Input: dimensioned drawing with shaded views. Units: mm. Origin: part minimum x, y, z. A direction names the side the tool comes from. Round coordinates to 2 decimals unless told otherwise and drop trailing zeros. Write each loop counter-clockwise with the first axis right and the second up, starting at its lowest first coordinate (ties: lowest second). Pieces come first, ordered by that corner, then holes. Notation, with made-up numbers: M 30,-24.75 L 75,-24.75 A19 ccw 75,-10.75 Z; hole C 66.25,-39 d10. An arc over 180 degrees is marked long. Put each result on its own line as item: value. Start each with the question number.
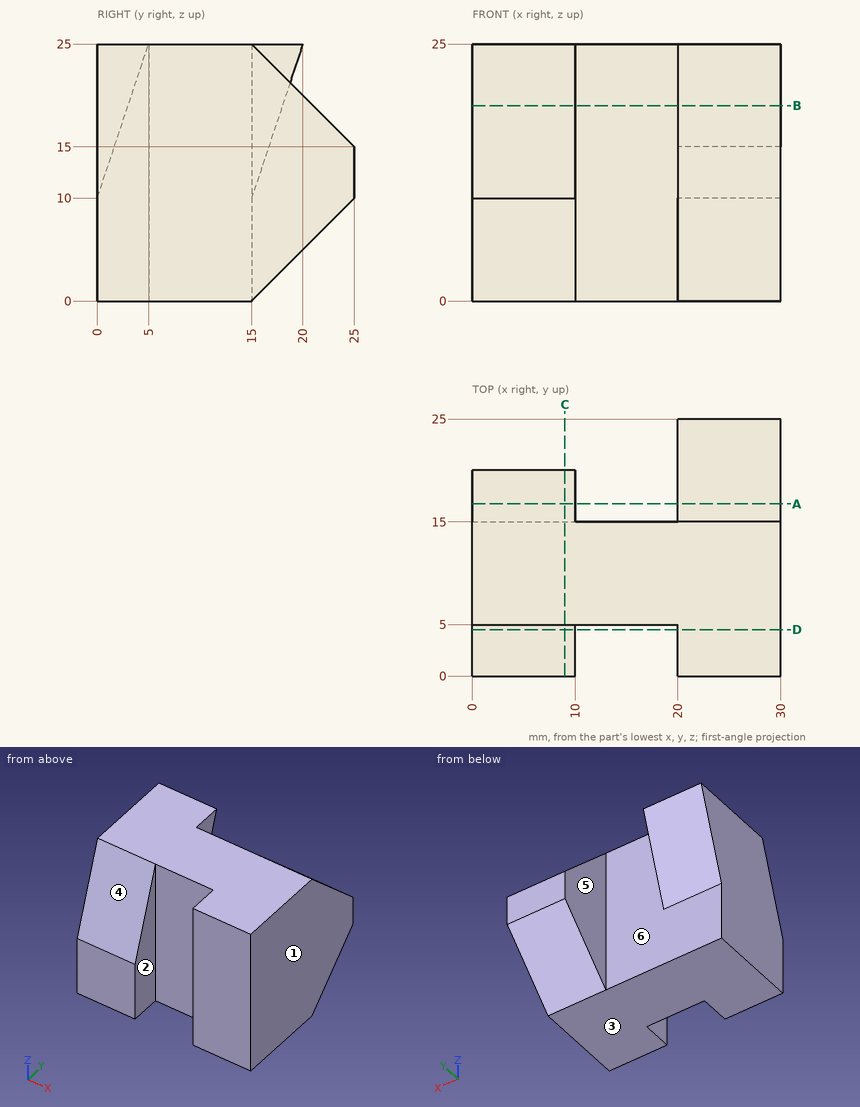
1) Section A-A, the plane y = 16.75. Output: boundary loops of the cut face in (x, z).
2) Section C-C, the plane x = 9. Output: boundary loops of the cut face in (y, z).
3) First-contact query: pin 1 (1 mm diameter, centred on x = 8, z = 22, fed in from +Y). Flat tip, straight axial feed; report the tip coordinate or a pass-through.
4) Section B-B, the plane z = 19. Output: boundary loops of the cut face in (x, y), and give its area (3 significant figures).
5) Ray query, probe 1 along Y at (x, z) = (11.5, 12.5); probe 2 along Z at (x, y) = (24, 18.75); probe 3 along Y at (x, z) = (5.75, 23). Return the intervals inside material, ascending.
6) Draft query along X for the marked faces 1, 2 and 3. Return one class per face: +X half, -X half, draft (parallel to the pull), parting line (faces both ways), or undercut.
7) Section D-D, the plane y = 4.5. Output: boundary loops of the cut face in (x, z).
8) Access query for the marked faces 4, 5 and 6. Directions: +Z, -Z, +X, -X, +Y, -Y. A direction counts if a zero-diameter tool reaches every point of the face in a straight line with its end or side. Return the directions, or none.
Solved:
1. outline: M 0,15.25 L 10,15.25 L 10,25 L 0,25 Z; M 20,1.75 L 30,1.75 L 30,23.25 L 20,23.25 Z
2. outline: M 0,0 L 15,0 L 15,10 L 20,25 L 5,25 L 0,10 Z
3. pin 1: stops at y = 19.17
4. outline: M 0,3 L 10,3 L 10,5 L 20,5 L 20,0 L 30,0 L 30,21 L 20,21 L 20,15 L 10,15 L 10,18 L 0,18 Z
4. area: 460 mm2
5. probe 1: y = 5 to 15
5. probe 2: z = 3.75 to 21.25
5. probe 3: y = 4.33 to 19.33
6. face 1: +X half
6. face 2: undercut
6. face 3: draft
7. outline: M 0,0 L 10,0 L 10,23.5 L 0,23.5 Z; M 20,0 L 30,0 L 30,25 L 20,25 Z
8. face 4: +Z, -X, -Y
8. face 5: +Z, -Z, +Y
8. face 6: -Z, +Y
